from build123d import *

# Parameters (mm, degrees)
SKETCH1_R           = 5
BOSS_EXTRUDE1_DEPTH = 68.222637
SKETCH2_R           = 1.437105979
CUT_EXTRUDE1_DEPTH  = 69.588105377
CHAMFER1_SIZE       = 1.128455


with BuildPart() as part:
    # Sketch1 → Boss-Extrude1 (new body)
    with BuildSketch(Plane(origin=(0, 0, 0), x_dir=(1, 0, 0), z_dir=(0, 1, 0))):
        with Locations(Location((0, 0, 0), (0, 0, 270))):
            Circle(SKETCH1_R)
    extrude(amount=BOSS_EXTRUDE1_DEPTH)

    # Sketch2 → Cut-Extrude1 (cut, through all)
    with BuildSketch(Plane(origin=(0, 0, 0), x_dir=(1, 0, 0), z_dir=(0, 1, 0))):
        with Locations(Location((0, 0, 0), (0, 0, 270))):
            Circle(SKETCH2_R)
    extrude(amount=CUT_EXTRUDE1_DEPTH, mode=Mode.SUBTRACT)

    # Chamfer1
    chamfer1_edges = [part.edges().sort_by_distance(p)[0] for p in [
        (0, 0, -5),
        (0, 68.222637, -5),
    ]]
    chamfer(chamfer1_edges, length=CHAMFER1_SIZE)


solid = part.part
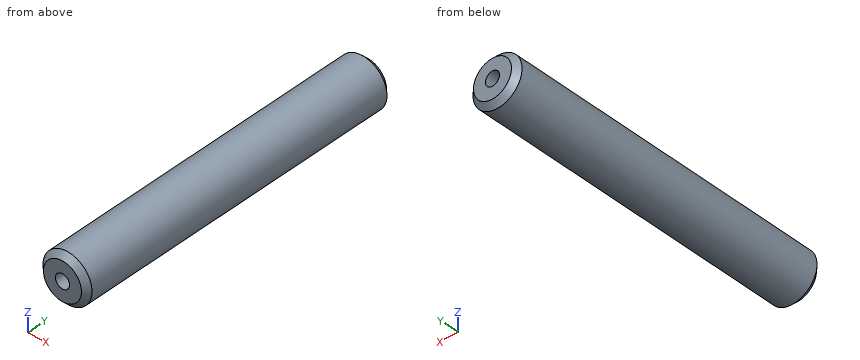
Design review of the part built by this model. Coordinates are the model's own, in mm. Coordinates: 2 decimals unless noted, no trailing zeros. Loops run counter-clockwise (first coordinate to the right, second up) from the corner with the lowest first, then second, coordinate; pieces in that order, holes last. Notation, with made-up numbers: (37, 47) -> (90, 47) arc R20 ccw to (90, 72) -> close; hole circle Ø3 at (36.25, 42.25). An arc over 180 degrees is marked (long way). Use a Markdown table: item, result. Add a question column.
Item 1: Clearance check with flat-ended pins moving along their axes: P1, Ø1, axis at x = 2.5, y = 44, coming from the +Z side; P2, Ø1, axis at x = -1.5, y = 47.5, coming from the +Z side. State where each tip first meets the part, or that it passes through.
Item 2: We need section A-A, the plane x = 0. Write out the cut boundary in (y, z), and give its area (3 significant figures).
Item 3: We need section C-C, the plane y = 11. Write out the cut boundary in (x, z).
Item 4: Wall thickness on L1, parallel to X at y = 39, z = 0; L2, parallel to Z at x = -1, y = 46; L3, parallel to Z at x = 0.75, y = 56: over which ranges is each line inside the solid? List them lowest first. Write a range as from..to.
Item 5: We need section B-B, the plane z = 0. Write out the cut boundary in (x, y).
Numbers:
| question | item | result |
|---|---|---|
| 1 | P1 | stops at z = 4.58 |
| 1 | P2 | stops at z = 4.9 |
| 2 | outline | (0, -3.87) -> (1.13, -5) -> (67.09, -5) -> (68.22, -3.87) -> (68.22, -1.44) -> (0, -1.44) -> close; (0, 1.44) -> (68.22, 1.44) -> (68.22, 3.87) -> (67.09, 5) -> (1.13, 5) -> (0, 3.87) -> close |
| 2 | area | 484 mm^2 |
| 3 | outline | circle Ø10 at (0, 0); hole circle Ø2.87 at (0, 0) |
| 4 | L1 | x = -5..-1.44, 1.44..5 |
| 4 | L2 | z = -4.9..-1.03, 1.03..4.9 |
| 4 | L3 | z = -4.94..-1.23, 1.23..4.94 |
| 5 | outline | (-5, 1.13) -> (-3.87, 0) -> (-1.44, 0) -> (-1.44, 68.22) -> (-3.87, 68.22) -> (-5, 67.09) -> close; (1.44, 0) -> (3.87, 0) -> (5, 1.13) -> (5, 67.09) -> (3.87, 68.22) -> (1.44, 68.22) -> close |
